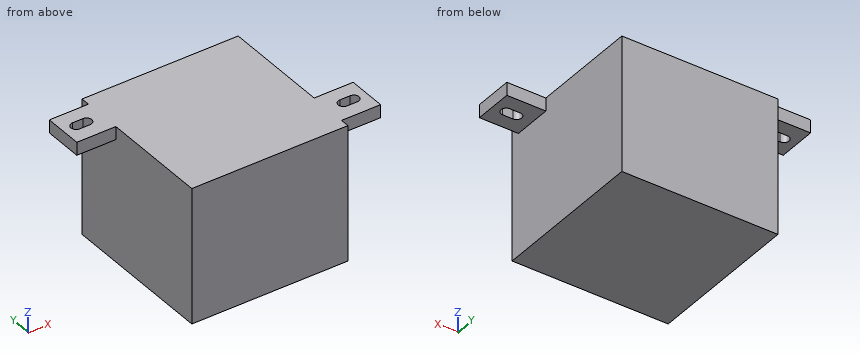
from build123d import *

# Parameters (mm, degrees)
SKETCH_1_W      = 60
SKETCH_1_H      = 60
EXTRUDE_1_DEPTH = 52
SKETCH_2_W      = 15
SKETCH_2_H      = 15
EXTRUDE_2_DEPTH = 5


with BuildPart() as part:
    # 草图1 → 凸台-拉伸1 (new body)
    with BuildSketch(Plane.XY):
        Rectangle(SKETCH_1_W, SKETCH_1_H)
    extrude(amount=EXTRUDE_1_DEPTH)

    # 草图2 → 凸台-拉伸2 (add)
    # profile 1 of 2: a face of its own
    with BuildSketch(Plane.XY.offset(52)):
        with Locations((-37.5, 19.032866311)):
            Rectangle(SKETCH_2_W, SKETCH_2_H)
        with BuildLine():
            Line((-40, 21.032866311), (-36, 21.032866311))
            ThreePointArc((-36, 21.032866311), (-34, 19.032866311), (-36, 17.032866311))
            Line((-36, 17.032866311), (-40, 17.032866311))
            ThreePointArc((-40, 17.032866311), (-42, 19.032866311), (-40, 21.032866311))
        make_face(mode=Mode.SUBTRACT)
    # profile 2 of 2: a face of its own
    with BuildSketch(Plane.XY.offset(52)):
        with Locations((37.5, -19.032866311)):
            Rectangle(SKETCH_2_W, SKETCH_2_H)
        with BuildLine():
            Line((40, -21.032866311), (36, -21.032866311))
            ThreePointArc((36, -21.032866311), (34, -19.032866311), (36, -17.032866311))
            Line((36, -17.032866311), (40, -17.032866311))
            ThreePointArc((40, -17.032866311), (42, -19.032866311), (40, -21.032866311))
        make_face(mode=Mode.SUBTRACT)
    extrude(amount=-EXTRUDE_2_DEPTH)


solid = part.part
For this review, take the finished solid that the model builds, in its own axes (mm). Coordinates: 2 decimals unless noted, no trailing zeros. Order: outer loops, then holes, each group sorted by start corner. A loop starts at its lowest first (then second) coordinate and runs counter-clockwise, first axis right, second up. Notation, with made-up numbers: (-11.5, 47.5) - (31.5, 47.5) arc R20 ccw to (31.5, 60.5) - close; hole circle Ø1 at (-19, 58.5). An arc over 180 degrees is marked (long way). Use one line per item in the form item = value.
Q1. Consider section C-C (z = 22.5). Give the boundary of the cut face in (x, y), then the cut area to 3 significant figures.
Checked values:
outline = (-30, -30) - (30, -30) - (30, 30) - (-30, 30) - close
area = 3,600 mm2
Q2. For P1, Ø1.2, axis at x = -38.5, z = 48.5, coming from the +Y side; P2, Ø4.5, axis at x = 38.5, z = 49.5, coming from the -Y side; P3, Ø15.5, axis at y = 12, z = 28, coming from the +X side, all flat-tipped, find the tip position at first contact; note any pin that passes through.
Checked values:
P1 = 26.53
P2 = -26.53
P3 = 30
Q3. Consider section B-B (y = 13.5). Give the boundary of the cut face in (x, z), then the cut area to 4 significant figures.
Checked values:
outline = (-45, 47) - (-30, 47) - (-30, 0) - (30, 0) - (30, 52) - (-45, 52) - close
area = 3,195 mm2
Q4. Consider section A-A (x = 38.5). Give the boundary of the cut face in (y, z).
Checked values:
outline = (-26.53, 47) - (-21.03, 47) - (-21.03, 52) - (-26.53, 52) - close; (-17.03, 47) - (-11.53, 47) - (-11.53, 52) - (-17.03, 52) - close
Q5. For probe 1 along X at (y, z) = (26.5, 32); probe 2 along Z at (x, y) = (-37, 23); probe 3 along X at (y, z) = (15, 50), list the stretches that pass through material, from the lowest coordinate up. Write a range as from..to.
Checked values:
probe_1 = -30..30
probe_2 = 47..52
probe_3 = -45..30
